Geometry: final body of the model. Coordinates: model frame, mm. Round coordinates to 2 decimals unless told otherwise and drop trailing zeros. Order: outer loops, then holes, each group sorted by start corner. A loop starts at its lowest first (then second) coordinate and runs counter-clockwise, first axis right, second up. Notation, with made-up numbers: M 69,79.25 L 76,79.25 A22 ccw 76,102.25 Z; hole C 71,6 d1. An arc over 180 degrees is marked long. Put each result on its own line as item: value. Start each with the question number.
1) Section A-A, the plane x = -13. Return loops of the section in (y, z), then the cut area to 3 significant figures.
2) Section C-C, the plane z = 6. Return loops of the section in (x, y).
3) Section D-D, the plane z = -7.5. Return loops of the section in (x, y), then the cut area to 3 significant figures.
4) First-contact query: P1, Ø10, axis at x = -15.5, z = 4, coming from the -Y side. Flat tip, straight axial feed; report the tip coordinate or a pass-through.
5) Section B-B, the plane y = -0.75. Return loops of the section in (x, z), then the cut area to 3 significant figures.
6) Material intervals for probe 1 along Z at (x, y) = (-14.5, -1.8); probe 2 along Z at (x, y) = (-15.5, -1.1); probe 3 along X at (y, z) = (-1.8, 5.5), sorted ascending. Write a range as [from, to].
from build123d import *

# Parameters (mm, degrees)
F1_DEPTH = 2.3622


with BuildPart() as f1:
    # F0 (on Front) → F1 (new body)
    with BuildSketch(Plane.XZ):
        with BuildLine():
            Line((-21.86199, -9.231923), (-14.44519, -9.231923))
            Line((-14.44519, -9.231923), (-14.44519, 1.702777))
            ThreePointArc((-14.44519, 1.702777), (-16.510649, 2.558318), (-17.36619, 4.623777))
            Line((-17.36619, 4.623777), (-30.06619, 4.623777))
            Line((-30.06619, 4.623777), (-21.86199, -9.231923))
        make_face()
        with BuildLine():
            Line((-14.44519, 1.702777), (-14.44519, -9.231923))
            Line((-14.44519, -9.231923), (-7.02839, -9.231923))
            Line((-7.02839, -9.231923), (1.17581, 4.623777))
            Line((1.17581, 4.623777), (-11.52419, 4.623777))
            ThreePointArc((-11.52419, 4.623777), (-12.379731, 2.558318), (-14.44519, 1.702777))
        make_face()
        with BuildLine():
            Line((-30.06619, 4.623777), (-17.36619, 4.623777))
            ThreePointArc((-17.36619, 4.623777), (-16.510649, 6.689236), (-14.44519, 7.544777))
            Line((-14.44519, 7.544777), (-14.44519, 18.479477))
            Line((-14.44519, 18.479477), (-21.86199, 18.479477))
            Line((-21.86199, 18.479477), (-30.06619, 4.623777))
        make_face()
        with BuildLine():
            ThreePointArc((-14.44519, 7.544777), (-12.379731, 6.689236), (-11.52419, 4.623777))
            Line((-11.52419, 4.623777), (1.17581, 4.623777))
            Line((1.17581, 4.623777), (-7.02839, 18.479477))
            Line((-7.02839, 18.479477), (-14.44519, 18.479477))
            Line((-14.44519, 18.479477), (-14.44519, 7.544777))
        make_face()
    extrude(amount=F1_DEPTH)


solid = f1.part
Result sheet:
1. outline: M -2.36,-9.23 L 0,-9.23 L 0,2.09 L -2.36,2.09 Z; M -2.36,7.16 L 0,7.16 L 0,18.48 L -2.36,18.48 Z
1. area: 53.5 mm2
2. outline: M -29.25,-2.36 L -17.02,-2.36 L -17.02,0 L -29.25,0 Z; M -11.87,-2.36 L 0.36,-2.36 L 0.36,0 L -11.87,0 Z
3. outline: M -22.89,-2.36 L -6,-2.36 L -6,0 L -22.89,0 Z
3. area: 39.9 mm2
4. P1: stops at y = -2.36
5. outline: M -30.07,4.62 L -21.86,-9.23 L -7.03,-9.23 L 1.18,4.62 L -7.03,18.48 L -21.86,18.48 Z; hole C -14.45,4.62 d5.84
5. area: 612 mm2
6. probe 1: z = [-9.23, 1.7], [7.54, 18.48]
6. probe 2: z = [-9.23, 1.9], [7.35, 18.48]
6. probe 3: x = [-29.55, -17.23], [-11.66, 0.66]
